```python
from build123d import *

# Parameters (mm, degrees)
SKETCH_1_R                   = 37
EXTRUDE_1_DEPTH              = 10
SKETCH_2_R                   = 22.5
EXTRUDE_2_DEPTH              = 54
SKETCH_3_R                   = 15
CUT_EXTRUDE_1_DEPTH          = 65
CUT_EXTRUDE_2_DEPTH          = 65
HOLE_WIZARD_M6_2_D           = 6.6
HOLE_WIZARD_M6_2_CBORE_D     = 11
HOLE_WIZARD_M6_2_CBORE_DEPTH = 6.5


with BuildPart() as part:
    # 草图1 → 凸台-拉伸1 (new body)
    with BuildSketch(Plane(origin=(0, 0, 0), x_dir=(0, 0, -1), z_dir=(1, 0, 0))):
        Circle(SKETCH_1_R)
    extrude(amount=EXTRUDE_1_DEPTH)

    # 草图2 → 凸台-拉伸2 (add)
    with BuildSketch(Plane(origin=(10, 0, 0), x_dir=(0, 0, -1), z_dir=(1, 0, 0))):
        Circle(SKETCH_2_R)
    extrude(amount=EXTRUDE_2_DEPTH)

    # 草图3 → 切除-拉伸1 (cut, through all)
    with BuildSketch(Plane.ZY):
        Circle(SKETCH_3_R)
    extrude(amount=-CUT_EXTRUDE_1_DEPTH, mode=Mode.SUBTRACT)

    # 草图6 → 切除-拉伸2 (cut, through all)
    with BuildSketch(Plane.ZY):
        with BuildLine():
            Line((-25.5, 26.809513237), (-25.5, -26.809513237))
            ThreePointArc((-25.5, -26.809513237), (-37, 0), (-25.5, 26.809513237))
        make_face()
        with BuildLine():
            Line((25.5, 26.809513237), (25.5, -26.809513237))
            ThreePointArc((25.5, -26.809513237), (37, 0), (25.5, 26.809513237))
        make_face()
    extrude(amount=-CUT_EXTRUDE_2_DEPTH, mode=Mode.SUBTRACT)

    # M6 六角头螺栓的柱形沉头孔2 (through all)
    with Locations(Plane.ZY):
        with Locations((-17.5, 24.5), (17.5, 24.5), (17.5, -24.5), (-17.5, -24.5)):
            CounterBoreHole(HOLE_WIZARD_M6_2_D / 2, HOLE_WIZARD_M6_2_CBORE_D / 2, HOLE_WIZARD_M6_2_CBORE_DEPTH)


solid = part.part
```
Check sheet for the modelled part. Datum: model origin and axes. Units: mm. A direction names the side the tool comes from. Give positions to 0.01 mm unless a question says otherwise; leave off trailing zeros. Order: outer loops, then holes, each group sorted by start corner. A loop starts at its lowest first (then second) coordinate and runs counter-clockwise, first axis right, second up. Notation, with made-up numbers: (71, 79.5) -> (108, 79.5) arc R18 cw to (108, 98.5) -> close; hole circle Ø10 at (-13.75, -6.5). An arc over 180 degrees is marked (long way). Use CSV: the item, a comma, the result in double quotes. Start each with the question number.
1) Go/stop test with flat-tipped pins: P1, Ø8, axis at y = 25.5, z = 20, coming from the +X side; P2, Ø1.5, axis at x = 50, z = 15.5, coming from the +Y side; P3, Ø6, axis at x = 35.5, y = 8.5, coming from the +Z side; P4, Ø3.5, axis at y = 25, z = -17, coming from the -X side. Record where each tip stops, or that it passes through.
2) Sectioned sample at B-B, the plane z = 0. Record the boundary of the cut face in (x, y), plus the area to 3 significant figures.
3) Set-up check for faces 4 (the face through (8.274, -26.508, 20.119)), 5 (the face through (36.622, -19.961, -10.382)), 6 (the face through (6.5, 22, -15)): record each of +Z, -Z, +X, -X, +Y, -Y from which the full face is reachable in a straight line by a thin tool's end or side.
4) Sectioned sample at C-C, the plane z = 17.5. Record the boundary of the cut face in (x, y), plus the area to 3 significant figures.
5) Mould release check, pull along Z, two halves, no side actions. Record for faces 1 (the face through (6.5, -27, 20)), 2 (the face through (64, -5, -15)), 3 (the face through (5, 37, 0)): released by +Z, released by -Z, zero draft, split by the parting line, or undercut.
6) Material ranges on line 1 (Z direction, x = 2, y = 24); line 2 (Y direction, x = 5, z = 17.5); line 3 (Y direction, x = 7.7, z = 17.5), recorded low to high. Write a range as from..to.
7) Sectioned sample at D-D, the plane y = -24.5. Record the boundary of the cut face in (x, z), plus the area to 3 significant figures.
8) Sectioned sample at A-A, the plane y = 0. Record the boundary of the cut face in (x, z), plus the area to 3 significant figures.
Recorded:
1,P1,"x = 10"
1,P2,"y = 16.99"
1,P3,"z = 21.82"
1,P4,"through"
2,outline,"(0, -37) -> (10, -37) -> (10, -22.5) -> (64, -22.5) -> (64, -15) -> (0, -15) -> close; (0, 15) -> (64, 15) -> (64, 22.5) -> (10, 22.5) -> (10, 37) -> (0, 37) -> close"
2,area,"1,250 mm2"
3,face 4,"+X, -X"
3,face 5,"+X"
3,face 6,"-X"
4,outline,"(0, -32.6) -> (10, -32.6) -> (10, -27.8) -> (6.5, -27.8) -> (6.5, -30) -> (0, -30) -> close; (0, -19) -> (6.5, -19) -> (6.5, -21.2) -> (10, -21.2) -> (10, -14.14) -> (64, -14.14) -> (64, 14.14) -> (10, 14.14) -> (10, 21.2) -> (6.5, 21.2) -> (6.5, 19) -> (0, 19) -> close; (0, 30) -> (6.5, 30) -> (6.5, 27.8) -> (10, 27.8) -> (10, 32.6) -> (0, 32.6) -> close"
4,area,"1,990 mm2"
5,face 1,"undercut"
5,face 2,"zero draft"
5,face 3,"split by the parting line"
6,line 1,"-25.5..-22.98, -12.02..12.02, 22.98..25.5"
6,line 2,"-32.6..-30, -19..19, 30..32.6"
6,line 3,"-32.6..-27.8, -21.2..21.2, 27.8..32.6"
7,outline,"(0, -25.5) -> (10, -25.5) -> (10, -20.8) -> (6.5, -20.8) -> (6.5, -23) -> (0, -23) -> close; (0, -12) -> (6.5, -12) -> (6.5, -14.2) -> (10, -14.2) -> (10, 14.2) -> (6.5, 14.2) -> (6.5, 12) -> (0, 12) -> close; (0, 23) -> (6.5, 23) -> (6.5, 20.8) -> (10, 20.8) -> (10, 25.5) -> (0, 25.5) -> close"
7,area,"321 mm2"
8,outline,"(0, -25.5) -> (10, -25.5) -> (10, -22.5) -> (64, -22.5) -> (64, -15) -> (0, -15) -> close; (0, 15) -> (64, 15) -> (64, 22.5) -> (10, 22.5) -> (10, 25.5) -> (0, 25.5) -> close"
8,area,"1,020 mm2"
